Design review of the part built by this model. Coordinates are the model's own, in mm. Face numbers are marked on the shaded views. A direction names the side the tool comes from. Round coordinates to 2 decimals unless told otherwise and drop trailing zeros. Write each loop counter-clockwise with the first axis right and the second up, starting at its lowest first coordinate (ties: lowest second). Pieces come first, ordered by that corner, then holes. Notation, with made-up numbers: (8, 30.25) - (45, 30.25) arc R28 ccw to (45, 59.25) - close; hole circle Ø1 at (47.25, 61.25). An arc over 180 degrees is marked (long way). Use one line per item in the form item = value.
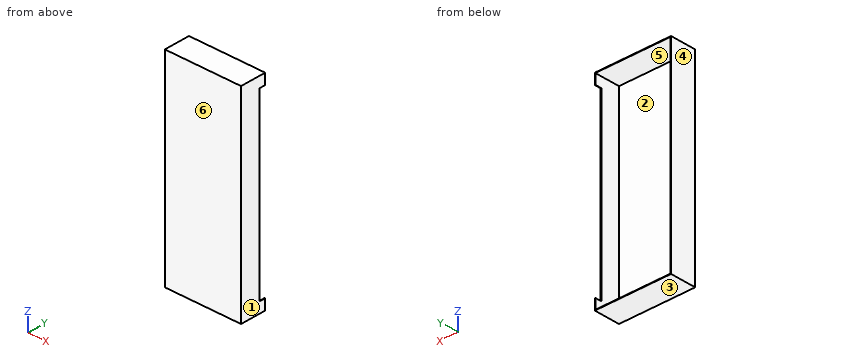
Autodesk Inventor part; units mm, degrees
ref_plane "YZ Plane" through (0, 0, 0) normal (1, 0, 0) x (0, 1, 0)
ref_plane "XZ Plane" through (0, 0, 0) normal (0, 1, 0) x (-1, 0, 0)
ref_plane "XY Plane" through (0, 0, 0) normal (0, 0, 1) x (1, 0, 0)
sketch "Sketch2" plane through (0, 0, 0) normal (0, 1, 0) x (-1, 0, 0)
  line L0 (0, 0) -> (914.4, 0)
  line L1 (914.4, 0) -> (914.4, -2438.4)
  line L2 (914.4, -2438.4) -> (0, -2438.4)
  line L3 (0, -2438.4) -> (0, 0)
  dimension "d22" = 2438.4
  dimension "d23" = 914.4
extrude "Extrusion2" add sketch "Sketch2" along normal blind 6.35
sketch "Sketch3" plane through (0, 6.35, 0) normal (0, 1, 0) x (1, 0, 0)
  line L0 (-914.4, 2438.4) -> (-914.4, 0)
  line L1 (0, 2438.4) -> (-914.4, 2438.4)
  line L2 (-914.4, 0) -> (0, 0)
  line L3 (0, 0) -> (0, 2438.4)
  line L4 (0, 2438.4) -> (-914.4, 2438.4)
  line L5 (-914.4, 2438.4) -> (-914.4, 0)
  line L6 (-6.35, 6.35) -> (-908.05, 6.35)
  line L7 (-908.05, 6.35) -> (-908.05, 2432.05)
  line L8 (-908.05, 2432.05) -> (-6.35, 2432.05)
  line L9 (-6.35, 2432.05) -> (-6.35, 6.35)
  dimension "d24" = 6.35
extrude "Extrusion3" add sketch "Sketch3" along normal blind 304.8
sketch "Sketch4" plane through (0, 0, 0) normal (1, 0, 0) x (0, 0, -1)
  line L0 (0, 0) -> (0, 311.15)
  line L1 (2438.4, 0) -> (2438.4, 311.15)
  line L2 (0, 311.15) -> (2438.4, 311.15)
  line L3 (2438.4, 311.15) -> (2311.4, 311.15)
  line L4 (2432.05, 311.15) -> (6.35, 311.15)
  line L5 (0, 311.15) -> (127, 311.15)
  line L6 (127, 311.15) -> (127, 234.95)
  line L7 (127, 234.95) -> (2311.4, 234.95)
  line L8 (2311.4, 234.95) -> (2311.4, 311.15)
  dimension "d27" = 127
  dimension "d28" = 127
  dimension "d29" = 76.2
extrude "Extrusion4" cut sketch "Sketch4" against normal blind 50.8
properties part number "ElectricalBoard.ver2-1111-2020"
Q1. For P1, Ø1, axis at x = -127.5, z = -1354, coming from the +Y side; P2, Ø7, axis at x = -3.5, z = -1626, coming from the +Y side, all flat-tipped, find the tip position at first contact; note any pin that passes through.
Calculated:
P1 = 6.35
P2 = 234.95
Q2. We need section C-C on z = -2051.5. Write out the cut boundary in (x, y).
Calculated:
outline = (-914.4, 0) - (0, 0) - (0, 234.95) - (-6.35, 234.95) - (-6.35, 6.35) - (-908.05, 6.35) - (-908.05, 311.15) - (-914.4, 311.15) - close
Q3. Draft analysis for pull direction X (two halves, no side actions). For the marked faces 1, 2, 3 and 4, state which applies: released by +X, released by -X, zero draft, split by the parting line, or undercut.
Calculated:
face_1 = released by +X
face_2 = undercut
face_3 = zero draft
face_4 = released by -X
Q4. Machinability: for the marked faces 5 and 6, which of the approach directions +Z, -Z, +X, -X, +Y, -Y give a long, thin tool a straight path to every point of the face, cutting with its end or side? Answer none if there is none.
Calculated:
face_5 = +Y
face_6 = +Z, -Z, +X, -X, -Y
Q5. We need section A-A on x = -256.5. Write out the cut boundary in (y, z).
Calculated:
outline = (0, -2438.4) - (311.15, -2438.4) - (311.15, -2432.05) - (6.35, -2432.05) - (6.35, -6.35) - (311.15, -6.35) - (311.15, 0) - (0, 0) - close
Q6. To check wall thickness, follow line 1 along Z through (x, y) = (-317, 290); line 2 along X through (y, z) = (59.5, -1210); line 3 along Y through (x, z) = (-373.5, -1821). State the ranges of each line that lie inside material, in increasing order. Write a range as from..to.
Calculated:
line_1 = -2438.4..-2432.05, -6.35..0
line_2 = -914.4..-908.05, -6.35..0
line_3 = 0..6.35
Q7. We need section B-B on y = 140. Write out the cut boundary in (x, z), then the cut area to 3 significant figures.
Calculated:
outline = (-914.4, -2438.4) - (0, -2438.4) - (0, 0) - (-914.4, 0) - close; hole (-908.05, -2432.05) - (-6.35, -2432.05) - (-6.35, -6.35) - (-908.05, -6.35) - close
area = 42,400 mm2
